Geometry: final body of the model. Coordinates: model frame, mm. A direction names the side the tool comes from. Round coordinates to 2 decimals unless told otherwise and drop trailing zeros. Loops run counter-clockwise (first coordinate to the right, second up) from the corner with the lowest first, then second, coordinate; pieces in that order, holes last. Notation, with made-up numbers: (-4, 20.25) - (3, 20.25) arc R14 ccw to (3, 39.25) - close; hole circle Ø11 at (31.25, -32). An arc over 180 degrees is marked (long way). Answer as CSV lines item,"result".
from build123d import *

# Parameters (mm, degrees)
F0_W     = 40.3748353374
F0_H     = 100
F1_DEPTH = 3
F3_D     = 3
F5_R     = 10
F7_DEPTH = 31.1417784542


with BuildPart() as f1:
    # F0 (on Top) → F1 (new body)
    with BuildSketch(Plane.XY):
        with Locations((20.1874176687, 50)):
            Rectangle(F0_W, F0_H)
    extrude(amount=F1_DEPTH)

    # F3 (through all)
    with Locations(Plane(origin=(0, 0, 0), x_dir=(1, 0, 0), z_dir=(0, 0, -1))):
        with Locations((10.3748353374, -25), (10.3748353374, -50)):
            Hole(F3_D / 2)

    # F5
    f5_edges = [f1.edges().sort_by_distance(p)[0] for p in [
        (40.374835, 100, 1.5),
        (40.374835, 0, 1.5),
    ]]
    fillet(f5_edges, radius=F5_R)

    # F6 (on face) → F7 (cut)
    with BuildSketch(Plane.XY.offset(3)):
        with BuildLine():
            ThreePointArc((27.8748353374, 20), (30.3748353374, 17.5), (32.8748353374, 20))
            Line((32.8748353374, 20), (32.8748353374, 60))
            ThreePointArc((32.8748353374, 60), (30.3748353374, 62.5), (27.8748353374, 60))
            Line((27.8748353374, 60), (27.8748353374, 20))
        make_face()
    extrude(amount=-F7_DEPTH, mode=Mode.SUBTRACT)

    # F8: F1 across plane


with BuildPart() as f1_1:
    add(f1.part)
    add(f1.part.mirror(Plane.YZ))


solid = f1_1.part
(1) Access query for faces 1 (the face through (-27.875, 40, 2)), 2 (the face through (1, 51, 3)). Directions: +Z, -Z, +X, -X, +Y, -Y. A direction counts if a zero-diameter tool reaches every point of the face in a straight line with its end or side. Return the directions, or none.
Findings below:
face 1,"+Z, -Z"
face 2,"+Z, +X, -X, +Y, -Y"
(2) Draft query along X for faces 3 (the face through (37.368, 2.852, 1.521)), 4 (the face through (-40.375, 49, 1)), 5 (the face through (-32.875, 40, 2)), 6 (the face through (32.875, 40, 2)). Return one class per face: pulls with the +X half, pulls with the -X half, needs draft (parallel to the pull), parting line crosses it, or undercut.
Findings below:
face 3,"pulls with the +X half"
face 4,"pulls with the -X half"
face 5,"undercut"
face 6,"undercut"
(3) Section A-A (z = 1.45). Output: boundary loops of the cut face in (x, y).
Findings below:
outline,"(-40.37, 10) arc R10 ccw to (-30.37, 0) - (30.37, 0) arc R10 ccw to (40.37, 10) - (40.37, 90) arc R10 ccw to (30.37, 100) - (-30.37, 100) arc R10 ccw to (-40.37, 90) - close; hole (-32.87, 20) arc R2.5 ccw to (-27.87, 20) - (-27.87, 60) arc R2.5 ccw to (-32.87, 60) - close; hole circle Ø3 at (-10.37, 25); hole circle Ø3 at (-10.37, 50); hole circle Ø3 at (10.37, 25); hole circle Ø3 at (10.37, 50); hole (27.87, 20) arc R2.5 ccw to (32.87, 20) - (32.87, 60) arc R2.5 ccw to (27.87, 60) - close"
(4) Material intervals for line 1 along X through (y, z) = (23, 0.7); line 2 along X through (y, z) = (25, 1.55); line 3 along Y through (x, z) = (10.5, 1.05), sorted ascending.
Findings below:
line 1,"-40.37 to -32.87, -27.87 to 27.87, 32.87 to 40.37"
line 2,"-40.37 to -32.87, -27.87 to -11.87, -8.87 to 8.87, 11.87 to 27.87, 32.87 to 40.37"
line 3,"0 to 23.51, 26.49 to 48.51, 51.49 to 100"
(5) Section C-C (x = -31.5). Output: boundary loops of the cut face in (y, z), and give its area (3 significant figures).
Findings below:
outline,"(0.06, 0) - (17.77, 0) - (17.77, 3) - (0.06, 3) - close; (62.23, 0) - (99.94, 0) - (99.94, 3) - (62.23, 3) - close"
area,"166 mm2"
(6) Section B-B (y = 25). Output: boundary loops of the cut face in (x, z), and give its area (3 significant figures).
Findings below:
outline,"(-40.37, 0) - (-32.87, 0) - (-32.87, 3) - (-40.37, 3) - close; (-27.87, 0) - (-11.87, 0) - (-11.87, 3) - (-27.87, 3) - close; (-8.87, 0) - (8.87, 0) - (8.87, 3) - (-8.87, 3) - close; (11.87, 0) - (27.87, 0) - (27.87, 3) - (11.87, 3) - close; (32.87, 0) - (40.37, 0) - (40.37, 3) - (32.87, 3) - close"
area,"194 mm2"
